from build123d import *

# Parameters (mm, degrees)
BOSS_EXTRUDE1_DEPTH      = 180.975
BOSS_EXTRUDE1_DEPTH_BACK = 180.975
SKETCH1_R                = 14.2875
CUT_EXTRUDE1_DEPTH       = 95.25
CUT_EXTRUDE1_DEPTH_BACK  = 95.25
SKETCH2_OUTSIDE_W        = 103.416
SKETCH2_OUTSIDE_H        = 103.416
SKETCH2_OUTSIDE_R        = 12.7
CUT_EXTRUDE2_DEPTH       = 131.191
CUT_EXTRUDE2_DEPTH_BACK  = 131.191
SKETCH3_OUTSIDE_W        = 103.416
SKETCH3_OUTSIDE_H        = 103.416
SKETCH3_OUTSIDE_R        = 13.6525
SKETCH5_OUTSIDE_W        = 103.416
SKETCH5_OUTSIDE_H        = 103.416
CUT_EXTRUDE4_DEPTH       = 35.941
CUT_EXTRUDE7_START       = 35.941
SKETCH6_R                = 14.2875
CUT_EXTRUDE7_DEPTH       = 35.941
SKETCH7_R                = 9.525
BOSS_EXTRUDE2_DEPTH      = 19.05


with BuildPart() as part:
    # Sketch1 → Boss-Extrude1 (new, two sides: drawn at the far end of the back side and taken through both)
    with BuildSketch(Plane(origin=(0, 0, 0), x_dir=(1, 0, 0), z_dir=(0, 1, 0)).offset(-BOSS_EXTRUDE1_DEPTH_BACK)):
        with Locations(Location((0, 0, 0), (0, 0, 270))):
            Circle(SKETCH1_R)
    extrude(amount=BOSS_EXTRUDE1_DEPTH + BOSS_EXTRUDE1_DEPTH_BACK)

    # Sketch2 outside → Cut-Extrude1 (cut, two sides: drawn at the far end of the back side and taken through both)
    with BuildSketch(Plane(origin=(0, 0, 0), x_dir=(1, 0, 0), z_dir=(0, 1, 0)).offset(-CUT_EXTRUDE1_DEPTH_BACK)):
        Rectangle(SKETCH2_OUTSIDE_W, SKETCH2_OUTSIDE_H)
        with Locations(Location((0, 0, 0), (0, 0, 270))):
            Circle(SKETCH2_OUTSIDE_R, mode=Mode.SUBTRACT)
    extrude(amount=CUT_EXTRUDE1_DEPTH + CUT_EXTRUDE1_DEPTH_BACK, mode=Mode.SUBTRACT)

    # Sketch3 outside → Cut-Extrude2 (cut, two sides: drawn at the far end of the back side and taken through both)
    with BuildSketch(Plane(origin=(0, 0, 0), x_dir=(1, 0, 0), z_dir=(0, 1, 0)).offset(-CUT_EXTRUDE2_DEPTH_BACK)):
        Rectangle(SKETCH3_OUTSIDE_W, SKETCH3_OUTSIDE_H)
        with Locations(Location((0, 0, 0), (0, 0, 270))):
            Circle(SKETCH3_OUTSIDE_R, mode=Mode.SUBTRACT)
    extrude(amount=CUT_EXTRUDE2_DEPTH + CUT_EXTRUDE2_DEPTH_BACK, mode=Mode.SUBTRACT)

    # Sketch5 outside → Cut-Extrude4 (cut)
    with BuildSketch(Plane(origin=(0, -131.191, 0), x_dir=(1, 0, 0), z_dir=(0, 1, 0))):
        Rectangle(SKETCH5_OUTSIDE_W, SKETCH5_OUTSIDE_H)
        with BuildLine():
            Line((0, -13.6525), (0, -13.5509))
            ThreePointArc((0, -13.5509), (-1.267011069, -13.491537116), (-2.522921262, -13.313968571))
            Line((-2.522921262, -13.313968571), (-2.54183726, -13.413792141))
            ThreePointArc((-2.54183726, -13.413792141), (-6.381040136, -12.069510472), (-9.65377533, -9.65377533))
            Line((-9.65377533, -9.65377533), (-9.581933281, -9.581933281))
            ThreePointArc((-9.581933281, -9.581933281), (-10.435869502, -8.644045265), (-11.198372194, -7.630422729))
            Line((-11.198372194, -7.630422729), (-11.282333747, -7.687633021))
            ThreePointArc((-11.282333747, -7.687633021), (-13.046509451, -4.022355949), (-13.6525, 0))
            Line((-13.6525, 0), (-13.5509, 0))
            ThreePointArc((-13.5509, 0), (-13.491537116, 1.267011069), (-13.313968571, 2.522921262))
            Line((-13.313968571, 2.522921262), (-13.413792141, 2.54183726))
            ThreePointArc((-13.413792141, 2.54183726), (-12.069510472, 6.381040136), (-9.65377533, 9.65377533))
            Line((-9.65377533, 9.65377533), (-9.581933281, 9.581933281))
            ThreePointArc((-9.581933281, 9.581933281), (-8.644045265, 10.435869502), (-7.630422729, 11.198372194))
            Line((-7.630422729, 11.198372194), (-7.687633021, 11.282333747))
            ThreePointArc((-7.687633021, 11.282333747), (-4.022355949, 13.046509451), (0, 13.6525))
            Line((0, 13.6525), (0, 13.5509))
            ThreePointArc((0, 13.5509), (1.267011069, 13.491537116), (2.522921262, 13.313968571))
            Line((2.522921262, 13.313968571), (2.54183726, 13.413792141))
            ThreePointArc((2.54183726, 13.413792141), (6.381040136, 12.069510472), (9.65377533, 9.65377533))
            Line((9.65377533, 9.65377533), (9.581933281, 9.581933281))
            ThreePointArc((9.581933281, 9.581933281), (10.435869502, 8.644045265), (11.198372194, 7.630422729))
            Line((11.198372194, 7.630422729), (11.282333747, 7.687633021))
            ThreePointArc((11.282333747, 7.687633021), (13.046509451, 4.022355949), (13.6525, 0))
            Line((13.6525, 0), (13.5509, 0))
            ThreePointArc((13.5509, 0), (13.491537116, -1.267011069), (13.313968571, -2.522921262))
            Line((13.313968571, -2.522921262), (13.413792141, -2.54183726))
            ThreePointArc((13.413792141, -2.54183726), (12.069510472, -6.381040136), (9.65377533, -9.65377533))
            Line((9.65377533, -9.65377533), (9.581933281, -9.581933281))
            ThreePointArc((9.581933281, -9.581933281), (8.644045265, -10.435869502), (7.630422729, -11.198372194))
            Line((7.630422729, -11.198372194), (7.687633021, -11.282333747))
            ThreePointArc((7.687633021, -11.282333747), (4.022355949, -13.046509451), (0, -13.6525))
        make_face(mode=Mode.SUBTRACT)
    extrude(amount=CUT_EXTRUDE4_DEPTH, mode=Mode.SUBTRACT)

    # Sketch6 → Cut-Extrude7 (cut)
    with BuildSketch(Plane.XZ.offset(-131.191).offset(CUT_EXTRUDE7_START)):
        with Locations(Location((0, 0, 0), (0, 0, 90))):
            Circle(SKETCH6_R)
        with BuildLine():
            Line((-13.6525, 0), (-13.5509, 0))
            ThreePointArc((-13.5509, 0), (-13.491537116, -1.267011069), (-13.313968571, -2.522921262))
            Line((-13.313968571, -2.522921262), (-13.413792141, -2.54183726))
            ThreePointArc((-13.413792141, -2.54183726), (-12.069510472, -6.381040136), (-9.65377533, -9.65377533))
            Line((-9.65377533, -9.65377533), (-9.581933281, -9.581933281))
            ThreePointArc((-9.581933281, -9.581933281), (-8.644045265, -10.435869502), (-7.630422729, -11.198372194))
            Line((-7.630422729, -11.198372194), (-7.687633021, -11.282333747))
            ThreePointArc((-7.687633021, -11.282333747), (-4.022355949, -13.046509451), (0, -13.6525))
            Line((0, -13.6525), (0, -13.5509))
            ThreePointArc((0, -13.5509), (1.267011069, -13.491537116), (2.522921262, -13.313968571))
            Line((2.522921262, -13.313968571), (2.54183726, -13.413792141))
            ThreePointArc((2.54183726, -13.413792141), (6.381040136, -12.069510472), (9.65377533, -9.65377533))
            Line((9.65377533, -9.65377533), (9.581933281, -9.581933281))
            ThreePointArc((9.581933281, -9.581933281), (10.435869502, -8.644045265), (11.198372194, -7.630422729))
            Line((11.198372194, -7.630422729), (11.282333747, -7.687633021))
            ThreePointArc((11.282333747, -7.687633021), (13.046509451, -4.022355949), (13.6525, 0))
            Line((13.6525, 0), (13.5509, 0))
            ThreePointArc((13.5509, 0), (13.491537116, 1.267011069), (13.313968571, 2.522921262))
            Line((13.313968571, 2.522921262), (13.413792141, 2.54183726))
            ThreePointArc((13.413792141, 2.54183726), (12.069510472, 6.381040136), (9.65377533, 9.65377533))
            Line((9.65377533, 9.65377533), (9.581933281, 9.581933281))
            ThreePointArc((9.581933281, 9.581933281), (8.644045265, 10.435869502), (7.630422729, 11.198372194))
            Line((7.630422729, 11.198372194), (7.687633021, 11.282333747))
            ThreePointArc((7.687633021, 11.282333747), (4.022355949, 13.046509451), (0, 13.6525))
            Line((0, 13.6525), (0, 13.5509))
            ThreePointArc((0, 13.5509), (-1.267011069, 13.491537116), (-2.522921262, 13.313968571))
            Line((-2.522921262, 13.313968571), (-2.54183726, 13.413792141))
            ThreePointArc((-2.54183726, 13.413792141), (-6.381040136, 12.069510472), (-9.65377533, 9.65377533))
            Line((-9.65377533, 9.65377533), (-9.581933281, 9.581933281))
            ThreePointArc((-9.581933281, 9.581933281), (-10.435869502, 8.644045265), (-11.198372194, 7.630422729))
            Line((-11.198372194, 7.630422729), (-11.282333747, 7.687633021))
            ThreePointArc((-11.282333747, 7.687633021), (-13.046509451, 4.022355949), (-13.6525, 0))
        make_face(mode=Mode.SUBTRACT)
    extrude(amount=-CUT_EXTRUDE7_DEPTH, mode=Mode.SUBTRACT)

    # Sketch7 → Boss-Extrude2 (add)
    with BuildSketch(Plane(origin=(0, 180.975, 0), x_dir=(1, 0, 0), z_dir=(0, 1, 0))):
        with Locations(Location((0, 0, 0), (0, 0, 90))):
            Circle(SKETCH7_R)
    extrude(amount=BOSS_EXTRUDE2_DEPTH)


solid = part.part
Geometry: final body of the model. Coordinates: model frame, mm. A direction names the side the tool comes from. Round coordinates to 2 decimals unless told otherwise and drop trailing zeros. Loops run counter-clockwise (first coordinate to the right, second up) from the corner with the lowest first, then second, coordinate; pieces in that order, holes last. Notation, with made-up numbers: (12.25, -30.75) -> (67.25, -30.75) arc R21 cw to (67.25, -2.75) -> close; hole circle Ø7 at (-13, 41). An arc over 180 degrees is marked (long way). One line per question, with ' | ' between items. Start each with the question number.
1. Section B-B on y = 42.5. Output: boundary loops of the cut face in (x, z), and give its area (3 significant figures).
2. Line query: line 1 along Y through (x, z) = (-12.5, 5.75) (3 decimals); line 2 along Y through (x, z) = (-9.25, -9) (3 decimals); line 3 along Y through (x, z) = (11.5, -2) (3 decimals). Output: solid intervals per line, ascending. Write a range as [from, to].
3. Set-up query: faces 4 (the face through (-12.096, -113.472, -6.33)), 5 (the face through (-9.3, 180.975, 3)), 6 (the face through (-13.03, -113.47, 4.08)). Return all of +Z, -Z, +X, -X, +Y, -Y with unobstructed straight access to the full face (end or side cutting, diameter ignored); none if empty.
4. Contact query for flat-ended pins moving along their axis: pin 1 (1 mm diameter, centred on x = 6, y = 6, fed in from -Z); pin 2 (1.5 mm diameter, centred on x = 0.5, y = -15, fed in from -Z); pin 3 (3 mm diameter, centred on y = 82.5, z = 10, fed in from +X). Output: stop coordinate, or through.
5. Section A-A on y = 148.5. Output: boundary loops of the cut face in (x, z) (1 decimal), and give its area (3 significant figures).
6. Mould query, pull axis Y, two halves, no side actions, for faces 1 (the face through (0.628, 155.735, -14.274)), 2 (the face through (0, 200.025, 0)), 3 (the face through (3.968, -113.472, 13.063)). Classes: pulls with the +Y half, pulls with the -Y half, needs draft (parallel to the pull), parting line crosses it, or undercut.
Returned:
1) outline: circle Ø25.4 at (0, 0) | area: 507 mm2
2) line 1: y = [-180.975, -131.191], [131.191, 180.975] | line 2: y = [-180.975, -95.25], [95.25, 180.975] | line 3: y = [-180.975, 180.975]
3) face 4: -Z, -X | face 5: +Y | face 6: +Z, -X
4) pin 1: stops at z = -11.45 | pin 2: stops at z = -12.7 | pin 3: stops at x = 9.44
5) outline: circle Ø28.6 at (0, 0) | area: 641 mm2
6) face 1: needs draft | face 2: pulls with the +Y half | face 3: undercut
